Work out the finished part from the listing and answer in its coordinate system (mm). Give positions to 0.01 mm unless a question says otherwise; leave off trailing zeros. Loops run counter-clockwise (first coordinate to the right, second up) from the corner with the lowest first, then second, coordinate; pieces in that order, holes last. Notation, with made-up numbers: (37.5, 15) -> (56.5, 15) arc R22 cw to (56.5, 33) -> close; hole circle Ø8 at (55.25, -28.5). An arc over 180 degrees is marked (long way). Answer as CSV lines item,"result". Start each with the question number.
1. Find the intervals of material crossed by line 1 along Y through (x, z) = (0, 0.9); line 2 along X through (y, z) = (-12, 1.7); line 3 along X through (y, z) = (36, 2.8), in increasing order.
2. Find section C-C, the plane x = 11.5. Give the vertices of the cut face in (y, z) (3 decimals), and give its area (3 significant figures).
3. Find section B-B, the plane z = 2.55. Give the vertices of the cut face in (x, y) (3 decimals), and give its area (3 significant figures).
4. Find section A-A, the plane x = -20. Give the vertices of the cut face in (y, z), and give its area (3 significant figures).
5. Find section D-D, the plane x = 30. Give the vertices of the cut face in (y, z).
from build123d import *

# Parameters (mm, degrees)
SKETCH_1_W          = 70
SKETCH_1_H          = 80
EXTRUDE_1_DEPTH     = 3
SKETCH_2_R          = 2.5
CUT_EXTRUDE_1_DEPTH = 10
SKETCH_3_R          = 1.5
CUT_EXTRUDE_2_DEPTH = 10
FILLET_1_R          = 10


with BuildPart() as part:
    # 草图1 → 凸台-拉伸1 (new body)
    with BuildSketch(Plane.XY):
        Rectangle(SKETCH_1_W, SKETCH_1_H)
    extrude(amount=EXTRUDE_1_DEPTH)

    # 草图2 → 切除-拉伸1 (cut)
    with BuildSketch(Plane(origin=(0, 0, 0), x_dir=(-1, 0, 0), z_dir=(0, 0, -1))):
        with Locations((-10.175, -9.825)):
            Circle(SKETCH_2_R)
    extrude(amount=-CUT_EXTRUDE_1_DEPTH, mode=Mode.SUBTRACT)

    # 草图3 → 切除-拉伸2 (cut)
    with BuildSketch(Plane.XY.offset(3)):
        with Locations((0, 30)):
            Circle(SKETCH_3_R)
        with Locations((20, 30)):
            Circle(SKETCH_3_R)
        with Locations((-20, 30)):
            Circle(SKETCH_3_R)
    extrude(amount=-CUT_EXTRUDE_2_DEPTH, mode=Mode.SUBTRACT)

    # 圆角1
    fillet_1_edges = [part.edges().sort_by_distance(p)[0] for p in [
        (35, -40, 1.5),
        (-35, -40, 1.5),
        (-35, 40, 1.5),
        (35, 40, 1.5),
    ]]
    fillet(fillet_1_edges, radius=FILLET_1_R)


solid = part.part
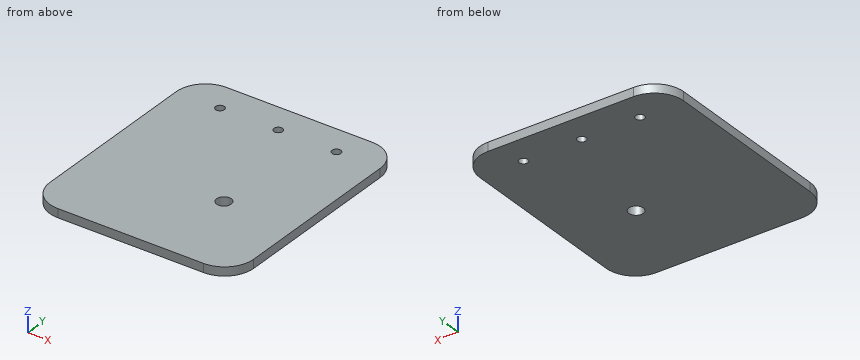
Resolved:
1,line 1,"y = -40 to 28.5, 31.5 to 40"
1,line 2,"x = -35 to 8.94, 11.41 to 35"
1,line 3,"x = -33 to 33"
2,outline,"(-40, 0) -> (-11.945, 0) -> (-11.945, 3) -> (-40, 3) -> close; (-7.705, 0) -> (40, 0) -> (40, 3) -> (-7.705, 3) -> close"
2,area,"227 mm^2"
3,outline,"(-35, -30) arc R10 ccw to (-25, -40) -> (25, -40) arc R10 ccw to (35, -30) -> (35, 30) arc R10 ccw to (25, 40) -> (-25, 40) arc R10 ccw to (-35, 30) -> close; hole circle Ø3 at (-20, 30); hole circle Ø3 at (0, 30); hole circle Ø5 at (10.175, -9.825); hole circle Ø3 at (20, 30)"
3,area,"5,470 mm^2"
4,outline,"(-40, 0) -> (28.5, 0) -> (28.5, 3) -> (-40, 3) -> close; (31.5, 0) -> (40, 0) -> (40, 3) -> (31.5, 3) -> close"
4,area,"231 mm^2"
5,outline,"(-38.66, 0) -> (38.66, 0) -> (38.66, 3) -> (-38.66, 3) -> close"
